```python
from build123d import *

# Parameters (mm, degrees)
DODANIE_WYCI_GNI_CIE1_DEPTH = 10
SZKIC2_R                    = 1.55
WYTNIJ_WYCI_GNI_CIE1_DEPTH  = 10
SZKIC3_W                    = 10
SZKIC3_H                    = 20
SZKIC3_H_2                  = 25
WYTNIJ_WYCI_GNI_CIE2_DEPTH  = 10
WYTNIJ_WYCI_GNI_CIE3_DEPTH  = 10
SZKIC5_W                    = 44.64499878
SZKIC5_H                    = 4
WYTNIJ_WYCI_GNI_CIE4_DEPTH  = 10


with BuildPart() as part:
    # Szkic1 → Dodanie-wyciągnięcie1 (new body)
    with BuildSketch(Plane.XY):
        with BuildLine():
            Line((-437.064585695, -68.955768861), (-437.064585695, -98.955768861))
            Line((-437.064585695, -98.955768861), (-437.064585695, -128.955768861))
            Line((-437.064585695, -128.955768861), (-447.064585695, -128.955768861))
            Line((-447.064585695, -128.955768861), (-467.064585695, -98.955768861))
            Line((-467.064585695, -98.955768861), (-498.66666852, -93.826601178))
            ThreePointArc((-498.66666852, -93.826601178), (-507.064585695, -83.955768861), (-498.66666852, -74.084936545))
            Line((-498.66666852, -74.084936545), (-467.064585695, -68.955768861))
            Line((-467.064585695, -68.955768861), (-437.064585695, -68.955768861))
        make_face()
    extrude(amount=DODANIE_WYCI_GNI_CIE1_DEPTH)

    # Szkic2 → Wytnij-wyciągnięcie1 (cut)
    with BuildSketch(Plane.XY.offset(10)):
        with Locations((-497.064585695, -83.955768861)):
            Circle(SZKIC2_R)
    extrude(amount=-WYTNIJ_WYCI_GNI_CIE1_DEPTH, mode=Mode.SUBTRACT)

    # Szkic3 → Wytnij-wyciągnięcie2 (cut)
    with BuildSketch(Plane(origin=(0, 0, 0), x_dir=(-1, 0, 0), z_dir=(0, 0, -1))):
        with Locations((442.064585695, -118.955768861)):
            Rectangle(SZKIC3_W, SZKIC3_H)
        with Locations((442.064585695, -81.455768861)):
            Rectangle(SZKIC3_W, SZKIC3_H_2)
    extrude(amount=-WYTNIJ_WYCI_GNI_CIE2_DEPTH, mode=Mode.SUBTRACT)

    # Szkic4 → Wytnij-wyciągnięcie3 (cut)
    with BuildSketch(Plane(origin=(0, 0, 0), x_dir=(-1, 0, 0), z_dir=(0, 0, -1))):
        Polygon((447.064585695, -78.955768861), (447.064585695, -82.055768861), (454.046285695, -82.055768861), (454.046285695, -83.430768861), (456.046285695, -83.430768861), (456.046285695, -82.055768861), (457.564585695, -82.055768861), (457.564585695, -78.955768861), (456.046285695, -78.955768861), (456.046285695, -77.580768861), (454.046285695, -77.580768861), (454.046285695, -78.955768861), align=None)
    extrude(amount=-WYTNIJ_WYCI_GNI_CIE3_DEPTH, mode=Mode.SUBTRACT)

    # Szkic5 → Wytnij-wyciągnięcie4 (cut)
    with BuildSketch(Plane(origin=(0, 0, 0), x_dir=(-1, 0, 0), z_dir=(0, 0, -1))):
        with Locations((469.387085085, -70.955768861)):
            Rectangle(SZKIC5_W, SZKIC5_H)
    extrude(amount=-WYTNIJ_WYCI_GNI_CIE4_DEPTH, mode=Mode.SUBTRACT)


solid = part.part
```
Input: part model. Units: mm. Frame: model coordinates. A direction names the side the tool comes from. Coordinates: 2 decimals unless noted, no trailing zeros. Write each loop counter-clockwise with the first axis right and the second up, starting at its lowest first coordinate (ties: lowest second). Pieces come first, ordered by that corner, then holes.
1) Section B-B on x = -442. Output: boundary loops of the cut face in (y, z).
2) Pin query (flat end, axial travel): pin 1 Ø0.7 at (y, z) = (-78.5, 7.5) entering from -X; pin 2 Ø5 at (x, y) = (-444, -89) entering from +Z; pin 3 Ø3.5 at (y, z) = (-81, 5.5) entering from +X; pin 4 Ø1 at (y, z) = (-118.5, 4.5) entering from -X. Return the tip coordinate at first contact, or that it passes through.
3) Section C-C on y = -80. Output: boundary loops of the cut face in (x, z), and give its area (3 significant figures).
4) Material intervals for line 1 along X through (y, z) = (-84, 6.25); line 2 along Y through (x, z) = (-442.5, 1.5); line 3 along Y through (x, z) = (-501.5, 3.25), sorted ascending.
5) Mould query, pull axis X, two halves, no side actions, for faces 1 (the flat face through (-442, -93.956, 5)), 2 (the flat face through (-447.065, -88, 5)), 3 (the flat face through (-455, -77.581, 5)), 4 (the flat face through (-456.046, -83, 5)). Classes: pulls with the +X half, pulls with the -X half, needs draft (parallel to the pull), parting line crosses it, or undercut.
6) Section A-A on z = 0.75. Output: boundary loops of the cut face in (x, y).
7) Set-up query: faces 5 (the flat face through (-442, -108.956, 5)), 6 (the flat face through (-451, -82.056, 5)), 7 (the flat face through (-447.065, -76, 5)). Return all of +Z, -Z, +X, -X, +Y, -Y with unobstructed straight access to the full face (end or side cutting, diameter ignored); none if empty.
Check result:
1. outline: (-108.96, 0) - (-93.96, 0) - (-93.96, 10) - (-108.96, 10) - close
2. pin 1: stops at x = -505.66
2. pin 2: passes through
2. pin 3: stops at x = -447.06
2. pin 4: stops at x = -454.37
3. outline: (-506.25, 0) - (-457.56, 0) - (-457.56, 10) - (-506.25, 10) - close
3. area: 487 mm2
4. line 1: x = -507.06 to -498.61, -495.52 to -447.06
4. line 2: y = -108.96 to -93.96
4. line 3: y = -92.92 to -74.99
5. face 1: needs draft
5. face 2: pulls with the +X half
5. face 3: undercut
5. face 4: undercut
6. outline: (-498.67, -93.83) - (-467.06, -98.96) - (-447.06, -128.96) - (-447.06, -108.96) - (-437.06, -108.96) - (-437.06, -93.96) - (-447.06, -93.96) - (-447.06, -82.06) - (-454.05, -82.06) - (-454.05, -83.43) - (-456.05, -83.43) - (-456.05, -82.06) - (-457.56, -82.06) - (-457.56, -78.96) - (-456.05, -78.96) - (-456.05, -77.58) - (-454.05, -77.58) - (-454.05, -78.96) - (-447.06, -78.96) - (-447.06, -72.96) - (-491.71, -72.96) - (-498.67, -74.08) arc R10 ccw to start; hole circle Ø3.1 at (-497.06, -83.96)
7. face 5: +Z, -Z, +X, -Y
7. face 6: +Z, -Z, +X
7. face 7: +Z, -Z, +X, +Y
